Check sheet for the modelled part. Datum: model origin and axes. Units: mm. Face numbers are marked on the shaded views. A direction names the side the tool comes from. Round coordinates to 2 decimals unless told otherwise and drop trailing zeros. Write each loop counter-clockwise with the first axis right and the second up, starting at its lowest first coordinate (ties: lowest second). Pieces come first, ordered by that corner, then holes. Notation, with made-up numbers: (-27.5, 7.5) - (-20.5, 7.5) arc R15 ccw to (-20.5, 13.5) - close; hole circle Ø1 at (-20, 44.5). An arc over 180 degrees is marked (long way). Answer as a JSON object with one key per item and string values. Group by question number.
Item 1: Gauge pin test, flat ends, axial feed: P1, Ø2, axis at y = 1, z = -20, coming from the +X side; P2, Ø0.8, axis at x = -3, z = 0.5, coming from the +Y side; P3, Ø3, axis at y = -1, z = -5, coming from the -X side; P4, Ø1, axis at x = 0.5, z = -1, coming from the -Y side. Record the tip position at first contact, or that the pin passes through.
Item 2: Set-up check for the marked faces 1 and 2: record each of +Z, -Z, +X, -X, +Y, -Y from which the full face is reachable in a straight line by a thin tool's end or side.
Item 3: Sectioned sample at C-C on z = 3.5. Record the boundary of the cut face in (x, y) (3 decimals).
Item 4: Sectioned sample at A-A on y = 0. Record the boundary of the cut face in (x, z) (3 decimals), plus the area to 3 significant figures.
Item 5: Sectioned sample at D-D on z = -10.5. Record the boundary of the cut face in (x, y).
Item 6: Thickness scan on line 1 (Z direction, x = -2.25, y = 1.15); line 2 (X direction, y = 1.35, z = -18); line 3 (Z direction, x = -1.5, y = 0.05). Record the ranges inside material, lowest first.
Item 7: Sectioned sample at B-B on x = 0. Record the boundary of the cut face in (y, z) (3 decimals), plus the area to 4 significant figures.
```python
from build123d import *

# Parameters (mm, degrees)
F3_DEPTH = 1.02
F2_R     = 0.24
F4_DEPTH = 25


with BuildPart() as f1:
    # F0 (on Front) → F1 (revolve)
    with BuildSketch(Plane.XZ):
        with BuildLine():
            Line((0, 0), (0, 5.33))
            Line((0, 5.33), (-2.165, 5.33))
            ThreePointArc((-2.165, 5.33), (-2.384203, 5.239203), (-2.475, 5.02))
            Line((-2.475, 5.02), (-2.475, 1.02))
            Line((-2.475, 1.02), (-2.92, 1.02))
            Line((-2.92, 1.02), (-2.92, 0))
            Line((-2.92, 0), (0, 0))
        make_face()
    revolve(axis=Axis((0, 0, 2.665), (0, 0, 1)))

    # F2 (on face) → F3 (join)
    with BuildSketch(Plane(origin=(0, 0, 0), x_dir=(1, 0, 0), z_dir=(0, 0, -1))):
        with BuildLine():
            ThreePointArc((-2.8608, -0.585), (-2.92, 0), (-2.8608, 0.585))
            Line((-2.8608, 0.585), (-4.0808, 0.585))
            Line((-4.0808, 0.585), (-4.0808, -0.585))
            Line((-4.0808, -0.585), (-2.8608, -0.585))
        make_face()
    extrude(amount=-F3_DEPTH)

    # F2 (on face) → F4 (join)
    with BuildSketch(Plane(origin=(0, 0, 0), x_dir=(1, 0, 0), z_dir=(0, 0, -1))):
        with Locations((-1.38125, 1.38125)):
            Circle(F2_R)
        with Locations((1.38125, 1.38125)):
            Circle(F2_R)
        with Locations((1.38125, -1.38125)):
            Circle(F2_R)
    extrude(amount=F4_DEPTH)


solid = f1.part
```
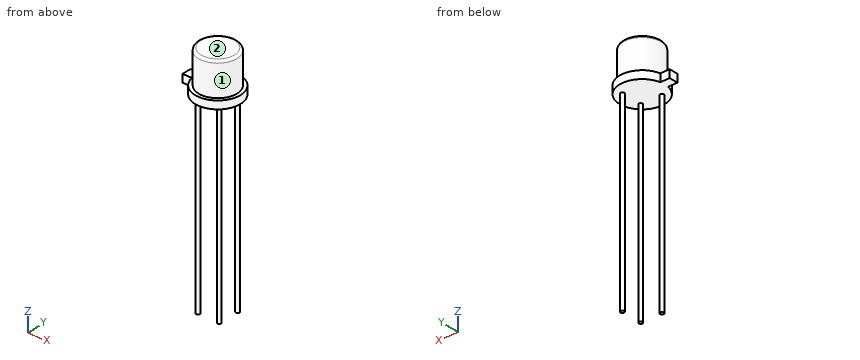
Completed:
{
 "1": {"P1": "x = 1.62", "P2": "y = 1.33", "P3": "x = -1.62", "P4": "through"},
 "2": {"face 1": "+Z", "face 2": "+Z, +X, -X, +Y, -Y"},
 "3": {"outline": "circle Ø4.95 at (0, 0)"},
 "4": {"outline": "(-4.081, 0) - (2.92, 0) - (2.92, 1.02) - (2.475, 1.02) - (2.475, 5.02) arc R0.31 ccw to (2.165, 5.33) - (-2.165, 5.33) arc R0.31 ccw to (-2.475, 5.02) - (-2.475, 1.02) - (-4.081, 1.02) - close", "area": "28.4 mm²"},
 "5": {"outline": "circle Ø0.48 at (-1.38, -1.38); circle Ø0.48 at (1.38, -1.38); circle Ø0.48 at (1.38, 1.38)"},
 "6": {"line 1": "0 to 1.02", "line 2": "1.14 to 1.62", "line 3": "0 to 5.33"},
 "7": {"outline": "(-2.92, 0) - (2.92, 0) - (2.92, 1.02) - (2.475, 1.02) - (2.475, 5.02) arc R0.31 ccw to (2.165, 5.33) - (-2.165, 5.33) arc R0.31 ccw to (-2.475, 5.02) - (-2.475, 1.02) - (-2.92, 1.02) - close", "area": "27.25 mm²"}
}
